Can you work these out from the model? Positions are in its coordinate system, mm. A direction names the side the tool comes from. Coordinates: 2 decimals unless noted, no trailing zeros. Order: outer loops, then holes, each group sorted by start corner. A loop starts at its lowest first (then second) coordinate and runs counter-clockwise, first axis right, second up. Notation, with made-up numbers: M 8,-12.5 L 22,-12.5 A25 cw 22,4.5 Z; hole C -14,5.25 d1. An arc over 180 degrees is marked long. Answer as CSV lines item,"result". Start each with the question number.
1. I need wall thicknesses on line 1 along Y through (x, z) = (-48, -40.5); line 2 along Y through (x, z) = (-105, 43); line 3 along Z through (x, y) = (100, -277.75). Which ranges of each line are inside material? Lowest first, please. Write a range as from..to.
2. On a 3-axis mill with a long thin cutter (end or side, diameter ignored), from which of +Z, -Z, +X, -X, +Y, -Y can I reach the whole of each face in a straight line? I mean faces 4 (the face through (-80.912, -279.043, 19.035)), 5 (the face through (76.65, -279.04, 32.16)), 6 (the face through (31.195, -279.043, -78.299)), 7 (the face through (54.27, -279.04, -62.96)). Say none if no direction works.
3. If we section it at B-B (x = -78.5): List the corners of the cut face in (y, z) for me, plus the area to 3 significant figures.
4. If we section it at D-D (z = 58.5): List the corners of the cut face in (x, y) for me, plus the area to 3 significant figures.
5. If we mould it in two halves opening along X, with no side actions, what happens to faces 1 (the face through (-64.827, -279.043, -53.864)), 2 (the face through (20.785, -279.043, 81.681)), 3 (the face through (-71.26, -279.04, 45.01))? For each: released by +X, released by -X, zero draft, split by the parting line, or undercut.
6. If we section it at A-A (z = -78): List the corners of the cut face in (x, y) for me, plus the area to 3 significant figures.
7. Will these pins go through, and if not, where does the flat tip stop? pin 1 (1 mm diameter, centred on x = -83, y = -278.5, fed in from -Z); pin 2 (8 mm diameter, centred on x = -49, z = 2.5, fed in from -Y); pin 3 (5 mm diameter, centred on x = -30, y = -275.5, fed in from +Z); pin 4 (1 mm diameter, centred on y = -277, z = -80, fed in from -X).
8. If we section it at C-C (x = 6): List the corners of the cut face in (y, z) for me, plus the area to 3 significant figures.
```python
from build123d import *

# Parameters (mm, degrees)
F3_DEPTH = 283.3549028797


with BuildPart() as f1:
    # F0 (on Top) → F1 (revolve)
    with BuildSketch(Plane.XY):
        with BuildLine():
            Line((0, -280.1789028797), (0, -283.3539028797))
            ThreePointArc((0, -283.3539028797), (63.5797243259, -281.7614157298), (127, -276.9879480051))
            Line((127, -276.9879480051), (127, -273.7969125493))
            ThreePointArc((127, -273.7969125493), (63.5801262199, -278.5823993082), (0, -280.1789028797))
        make_face()
    revolve(axis=Axis((0, -280.1789028797, 0), (0, -1, 0)))

    # F2 (on Front) → F3 (cut, through all)
    with BuildSketch(Plane.XZ):
        with BuildLine():
            ThreePointArc((-116.9396589005, 49.5390368924), (-123.7244866651, -28.6574841789), (-83.2507657642, -95.907820326))
            Line((-83.2507657642, -95.907820326), (-45.8795627998, -10.6267795528))
            Line((-45.8795627998, -10.6267795528), (-116.9396589005, 49.5390368924))
        make_face()
        with BuildLine():
            ThreePointArc((-83.2507657642, -95.907820326), (-10.9780819308, -126.5246288954), (65.4878560688, -108.8133296408))
            Line((65.4878560688, -108.8133296408), (-4.0708966587, -46.9179126428))
            Line((-4.0708966587, -46.9179126428), (-83.2507657642, -95.907820326))
        make_face()
        with BuildLine():
            ThreePointArc((65.4878560688, -108.8133296408), (110.5575816503, -62.4981690902), (127, 0))
            ThreePointArc((127, 0), (126.1784644986, 14.4220351119), (123.7244866651, 28.6574841789))
            Line((123.7244866651, 28.6574841789), (43.3636103, -18.3700851417))
            Line((43.3636103, -18.3700851417), (65.4878560688, -108.8133296408))
        make_face()
        with BuildLine():
            Line((30.871081699, 35.564575649), (123.7244866651, 28.6574841789))
            ThreePointArc((123.7244866651, 28.6574841789), (83.2507657642, 95.907820326), (10.9780819308, 126.5246288954))
            Line((10.9780819308, 126.5246288954), (30.871081699, 35.564575649))
        make_face()
        with BuildLine():
            Line((-24.2842325405, 40.3502016882), (10.9780819308, 126.5246288954))
            ThreePointArc((10.9780819308, 126.5246288954), (-65.4878560688, 108.8133296408), (-116.9396589005, 49.5390368924))
            Line((-116.9396589005, 49.5390368924), (-24.2842325405, 40.3502016882))
        make_face()
    extrude(amount=F3_DEPTH, mode=Mode.SUBTRACT)


solid = f1.part
```
Solved:
1,line 1,"-281.8..-278.62"
1,line 2,"-278.28..-275.09"
1,line 3,"14.77..30.42"
2,face 4,"-X, +Y, -Y"
2,face 5,"+Z, +X, +Y, -Y"
2,face 6,"-Z, +Y, -Y"
2,face 7,"+X, +Y, -Y"
3,outline,"M -280.81,16.99 L -277.63,16.99 A1264.39 cw -276.92,45.73 L -280.1,45.73 A1267.57 ccw Z; M -278.07,-85.07 A1267.57 ccw -277.51,-92.97 L -274.32,-92.97 A1264.39 cw -274.88,-85.07 Z"
3,area,"117 mm²"
4,outline,"M -16.86,-281.89 A1268.65 ccw 25.86,-281.74 L 25.86,-278.56 A1265.47 cw -16.86,-278.72 Z"
4,area,"136 mm²"
5,face 1,"released by -X"
5,face 2,"released by +X"
5,face 3,"undercut"
6,outline,"M -75.4,-278.71 A1267.6 ccw -54.31,-279.79 L -54.31,-276.61 A1264.42 cw -75.4,-275.53 Z; M 30.86,-280.58 A1267.6 ccw 57.95,-279.63 L 57.95,-276.45 A1264.42 cw 30.86,-277.4 Z"
6,area,"153 mm²"
7,pin 1,"z = 20.38"
7,pin 2,"y = -282.55"
7,pin 3,"through"
7,pin 4,"x = -76.5"
8,outline,"M -282.11,-55.88 L -278.93,-55.88 A1266.81 cw -274.99,114.36 L -278.18,114.36 A1269.99 ccw Z"
8,area,"541 mm²"
